Input: part model. Units: mm. Frame: model coordinates. Coordinates: 2 decimals unless noted, no trailing zeros. Write each loop counter-clockwise with the first axis right and the second up, starting at its lowest first coordinate (ties: lowest second). Pieces come first, ordered by that corner, then holes. Notation, with made-up numbers: (-36.75, 84.25) - (9.25, 84.25) arc R21 cw to (9.25, 101.25) - close; hole circle Ø11 at (-37.75, 8.25). An arc over 180 degrees is marked (long way). One line per question, with ' | ' between items. Start each with the question number.
1) First-contact query: P1, Ø1, axis at y = 1, z = -1, coming from the +X side; P2, Ø1, axis at x = 2, z = -0.5, coming from the +Y side; P3, Ø2, axis at x = 0, y = 0, coming from the -Z side. Flat tips, straight axial feed; report the tip coordinate or a pass-through.
2) Section query C-C on z = -1.3. Return loops of the section in (x, y), and give its area (3 significant figures).
3) Line query: line 1 (X direction, y = 0, z = -1.7); line 2 (Y direction, x = 0, z = -1.6); line 3 (X direction, y = 1.5, z = -1.45). Output: solid intervals per line, ascending.
4) Section query D-D on z = -0.2. Return loops of the section in (x, y).
5) Draft query along Y for faces 1 (the flat face through (-2, 0, -2.2)), 2 (the cylindrical face through (-0.1, 4.5, -1.9)), 3 (the conical face through (2.057, -0.648, -0.094)), 4 (the cylindrical face through (-1.216, -1.115, -1.085)). Return one class per face: released by +Y, released by -Y, zero draft, split by the parting line, or undercut.
6) Section query A-A on x = 0. Return loops of the section in (y, z), and give its area (3 significant figures).
7) Section query B-B on y = 0. Return loops of the section in (x, z).
```python
from build123d import *

# Parameters (mm, degrees)
SKETCH3_W          = 2.43419071
SKETCH3_H          = 7.16478775
CUT_EXTRUDE1_DEPTH = 3.2


with BuildPart() as part:
    # Sketch2 → Revolve1 (revolve)
    with BuildSketch(Plane(origin=(0, 0, 0), x_dir=(1, 0, 0), z_dir=(0, 1, 0))):
        Polygon((2, 0), (4.5, 1.502151548), (4.5, 2.2), (1.65, 2.2), (1.65, 0), align=None)
    revolve(axis=Axis((0, 0, 0), (0, 0, -1)))

    # Sketch3 → Cut-Extrude1 (cut, through all)
    with BuildSketch(Plane(origin=(0, 0, -2.2), x_dir=(-1, 0, 0), z_dir=(0, 0, -1))):
        with Locations((-5.217095355, -0.122475004)):
            Rectangle(SKETCH3_W, SKETCH3_H)
    cut_extrude1 = extrude(amount=-CUT_EXTRUDE1_DEPTH, mode=Mode.SUBTRACT)

    # Mirror1: Cut-Extrude1 across plane
    add(cut_extrude1.mirror(Plane(origin=(0, 0, 0), x_dir=(0, 0, 1), z_dir=(1, 0, 0))), mode=Mode.SUBTRACT)


solid = part.part
```
Answer key:
1) P1: x = 4 | P2: y = 3.12 | P3: through
2) outline: (-4, -1.16) arc R4.16 ccw to (4, -1.16) - (4, 1.16) arc R4.16 ccw to (-4, 1.16) - close; hole circle Ø3.3 at (0, 0) | area: 45.4 mm²
3) line 1: -4 to -1.65, 1.65 to 4 | line 2: -4.5 to -1.65, 1.65 to 4.5 | line 3: -4 to -0.69, 0.69 to 4
4) outline: circle Ø4.67 at (0, 0); hole circle Ø3.3 at (0, 0)
5) face 1: zero draft | face 2: released by +Y | face 3: split by the parting line | face 4: undercut
6) outline: (-4.5, -2.2) - (-1.65, -2.2) - (-1.65, 0) - (-2, 0) - (-4.5, -1.5) - close; (1.65, -2.2) - (4.5, -2.2) - (4.5, -1.5) - (2, 0) - (1.65, 0) - close | area: 8.78 mm²
7) outline: (-4, -2.2) - (-1.65, -2.2) - (-1.65, 0) - (-2, 0) - (-4, -1.2) - close; (1.65, -2.2) - (4, -2.2) - (4, -1.2) - (2, 0) - (1.65, 0) - close
